The listing builds one solid part. Answer for the finished solid, in the listing's coordinates (mm). A direction names the side the tool comes from. Give positions to 0.01 mm unless a question says otherwise; leave off trailing zeros. Order: outer loops, then holes, each group sorted by start corner. A loop starts at its lowest first (then second) coordinate and runs counter-clockwise, first axis right, second up. Notation, with made-up numbers: (-20, 68) - (-6, 68) arc R11 ccw to (-6, 76) - close; hole circle Ø2 at (18.5, 1). An arc over 180 degrees is marked (long way). Use CSV: the item, a comma, the result in double quotes.
```python
from build123d import *

# Parameters (mm, degrees)
BOSS_EXTRUDE1_DEPTH = 101.6
SKETCH2_R           = 13.49375
CUT_EXTRUDE1_DEPTH  = 228.6


with BuildPart() as part:
    # Sketch1 → Boss-Extrude1 (new body)
    with BuildSketch(Plane.XY):
        with BuildLine():
            Line((-16.637, -19.05), (16.637, -19.05))
            ThreePointArc((16.637, -19.05), (18.343248663, -18.343248663), (19.05, -16.637))
            Line((19.05, -16.637), (19.05, 16.637))
            ThreePointArc((19.05, 16.637), (18.343248663, 18.343248663), (16.637, 19.05))
            Line((16.637, 19.05), (-16.637, 19.05))
            ThreePointArc((-16.637, 19.05), (-18.343248663, 18.343248663), (-19.05, 16.637))
            Line((-19.05, 16.637), (-19.05, -16.637))
            ThreePointArc((-19.05, -16.637), (-18.343248663, -18.343248663), (-16.637, -19.05))
        make_face()
        with BuildLine():
            Line((-14.224, -16.637), (14.224, -16.637))
            ThreePointArc((14.224, -16.637), (15.930248663, -15.930248663), (16.637, -14.224))
            Line((16.637, -14.224), (16.637, 14.224))
            ThreePointArc((16.637, 14.224), (15.930248663, 15.930248663), (14.224, 16.637))
            Line((14.224, 16.637), (-14.224, 16.637))
            ThreePointArc((-14.224, 16.637), (-15.930248663, 15.930248663), (-16.637, 14.224))
            Line((-16.637, 14.224), (-16.637, -14.224))
            ThreePointArc((-16.637, -14.224), (-15.930248663, -15.930248663), (-14.224, -16.637))
        make_face(mode=Mode.SUBTRACT)
    extrude(amount=BOSS_EXTRUDE1_DEPTH)

    # Sketch2 → Cut-Extrude1 (cut, symmetric)
    with BuildSketch(Plane(origin=(0, 0, 0), x_dir=(1, 0, 0), z_dir=(0, 1, 0))):
        with Locations((0, -19.05)):
            Circle(SKETCH2_R)
    extrude(amount=CUT_EXTRUDE1_DEPTH, both=True, mode=Mode.SUBTRACT)


solid = part.part
```
Item 1: The part is cut by section A-A (y = -1.5). Give the vertices of the cut face in (x, z).
Taken from the geometry:
outline,"(-19.05, 0) - (-16.64, 0) - (-16.64, 101.6) - (-19.05, 101.6) - close; (16.64, 0) - (19.05, 0) - (19.05, 101.6) - (16.64, 101.6) - close"
Item 2: The part is cut by section C-C (x = 0). Give the vertices of the cut face in (y, z), and give its area (3 significant figures).
Taken from the geometry:
outline,"(-19.05, 0) - (-16.64, 0) - (-16.64, 5.56) - (-19.05, 5.56) - close; (-19.05, 32.54) - (-16.64, 32.54) - (-16.64, 101.6) - (-19.05, 101.6) - close; (16.64, 0) - (19.05, 0) - (19.05, 5.56) - (16.64, 5.56) - close; (16.64, 32.54) - (19.05, 32.54) - (19.05, 101.6) - (16.64, 101.6) - close"
area,"360 mm^2"
Item 3: The mould has two halves that part along Y. Classify faces 3 (the face through (-2.93, 17.86, 32.22)), 4 (the face through (-15.95, -15.91, 50.09)), 5 (the face through (18.362, 18.324, 50.089)): +Y half, -Y half, draft (parallel to the pull), parting line (faces both ways), or undercut.
Taken from the geometry:
face 3,"draft"
face 4,"undercut"
face 5,"+Y half"
Item 4: The part is cut by section D-D (z = 19.05). Give the vertices of the cut face in (x, y).
Taken from the geometry:
outline,"(-19.05, -16.64) arc R2.41 ccw to (-16.64, -19.05) - (-13.49, -19.05) - (-13.49, -16.64) - (-14.22, -16.64) arc R2.41 cw to (-16.64, -14.22) - (-16.64, 14.22) arc R2.41 cw to (-14.22, 16.64) - (-13.49, 16.64) - (-13.49, 19.05) - (-16.64, 19.05) arc R2.41 ccw to (-19.05, 16.64) - close; (13.49, -19.05) - (16.64, -19.05) arc R2.41 ccw to (19.05, -16.64) - (19.05, 16.64) arc R2.41 ccw to (16.64, 19.05) - (13.49, 19.05) - (13.49, 16.64) - (14.22, 16.64) arc R2.41 cw to (16.64, 14.22) - (16.64, -14.22) arc R2.41 cw to (14.22, -16.64) - (13.49, -16.64) - close"
Item 5: The part is cut by section B-B (z = 94.5). Give the vertices of the cut face in (x, y).
Taken from the geometry:
outline,"(-19.05, -16.64) arc R2.41 ccw to (-16.64, -19.05) - (16.64, -19.05) arc R2.41 ccw to (19.05, -16.64) - (19.05, 16.64) arc R2.41 ccw to (16.64, 19.05) - (-16.64, 19.05) arc R2.41 ccw to (-19.05, 16.64) - close; hole (-16.64, -14.22) arc R2.41 ccw to (-14.22, -16.64) - (14.22, -16.64) arc R2.41 ccw to (16.64, -14.22) - (16.64, 14.22) arc R2.41 ccw to (14.22, 16.64) - (-14.22, 16.64) arc R2.41 ccw to (-16.64, 14.22) - close"
Item 6: Find the intervals of material crossed by line 1 along X through (y, z) = (5, 38); line 2 along Z through (x, y) = (0, 17.5), in increasing order.
Taken from the geometry:
line 1,"-19.05 to -16.64, 16.64 to 19.05"
line 2,"0 to 5.56, 32.54 to 101.6"
Item 7: Which of the six approach directions +Z, -Z, +X, -X, +Y, -Y give full straight-line access (tool end or side, diameter ignored) to faces 1 (the face through (0, -19.05, 50)), 2 (the face through (15.95, 15.91, 50.09))?
Taken from the geometry:
face 1,"+Z, -Z, +X, -X, -Y"
face 2,"+Z, -Z"
